from build123d import *

# Parameters (mm, degrees)
F0_W     = 100
F0_H     = 50
F0_R     = 12.5
F1_DEPTH = 10
F2_W     = 10
F2_H     = 50
F3_DEPTH = 5
F5_DEPTH = 50.001
F6_R     = 2.5
F7_DEPTH = 10
F8_R     = 4.99999


# Not quite as in the source:
# - a fillet or chamfer is up to 0.001 mm smaller than in the source, because OpenCascade refuses the exact size


with BuildPart() as f1:
    # F0 (on Top) → F1 (new body)
    with BuildSketch(Plane.XY):
        Rectangle(F0_W, F0_H)
        Circle(F0_R, mode=Mode.SUBTRACT)
    extrude(amount=F1_DEPTH)

    # F2 (on face) → F3 (cut)
    with BuildSketch(Plane.XY.offset(10)):
        with Locations((-35, 0)):
            Rectangle(F2_W, F2_H)
        with BuildLine():
            Line((-7.5, -10), (-7.5, -25))
            Line((-7.5, -25), (7.5, -25))
            Line((7.5, -25), (7.5, -10))
            ThreePointArc((7.5, -10), (0, -12.5), (-7.5, -10))
        make_face()
        with BuildLine():
            Line((7.5, 25), (-7.5, 25))
            Line((-7.5, 25), (-7.5, 10))
            ThreePointArc((-7.5, 10), (0, 12.5), (7.5, 10))
            Line((7.5, 10), (7.5, 25))
        make_face()
    extrude(amount=-F3_DEPTH, mode=Mode.SUBTRACT)

    # F4 (on face) → F5 (cut, through all)
    with BuildSketch(Plane.XZ.offset(25)):
        Polygon((34.8284628647, 10), (19.8284628647, 10), (16.3643612496, 4), (38.2925644799, 4), align=None)
    extrude(amount=-F5_DEPTH, mode=Mode.SUBTRACT)

    # F6 (on face) → F7 (join)
    with BuildSketch(Plane.YZ.offset(50)):
        with Locations((0, 5)):
            Circle(F6_R)
    extrude(amount=F7_DEPTH)

    # F8 (radius 5 in the source; OpenCascade refuses exactly that, so slightly less here)
    f8_edges = [f1.edges().sort_by_distance(p)[0] for p in [
        (-18.75, -25, 10),
        (-18.75, 25, 10),
        (-7.5, -17.5, 10),
        (-7.5, 17.5, 10),
    ]]
    fillet(f8_edges, radius=F8_R)


solid = f1.part
Check sheet for the modelled part. Datum: model origin and axes. Units: mm. A direction names the side the tool comes from. Round coordinates to 2 decimals unless told otherwise and drop trailing zeros. Loops run counter-clockwise (first coordinate to the right, second up) from the corner with the lowest first, then second, coordinate; pieces in that order, holes last. Notation, with made-up numbers: (12, 83) - (48, 83) arc R16 ccw to (48, 105) - close; hole circle Ø6 at (31.25, -2). An arc over 180 degrees is marked (long way). Answer as CSV lines item,"result". Start each with the question number.
Item 1: Release check for a two-part mould opening along X. For faces 1 (the cylindrical face through (-19, -24, 8)), 2 (the flat face through (-45, 0, 10)), 3 (the flat face through (50, 0, 2)) record: +X half, -X half, draft (parallel to the pull), parting line (faces both ways), or undercut.
Item 2: Section check A-A (x = 0). Record the boundary of the cut face in (y, z), and give its area (3 significant figures).
Item 3: Section check D-D (y = 1.5). Record the boundary of the cut face in (x, z).
Item 4: Section check B-B (z = 1.5). Record the boundary of the cut face in (x, y), and give its area (3 significant figures).
Item 5: Depth check by flat-ended pin: P1, Ø5, axis at x = -34.5, y = 3, coming from the +Z side; P2, Ø6, axis at x = 5.5, y = 4.5, coming from the +Z side; P3, Ø1, axis at y = -4.5, z = 7, coming from the +X side. Enter the tip coordinate at first touch or a pass-through.
Item 6: Set-up check for faces 4 (the cylindrical face through (54.93, -0.33, 7.48)), 5 (the flat face through (-1, -25, 4)), 6 (the cylindrical face through (-19, 24, 8)), 7 (the flat face through (27, 0, 4)), 8 (the flat face through (-30, 0, 8)): record each of +Z, -Z, +X, -X, +Y, -Y from which the full face is reachable in a straight line by a thin tool's end or side.
Item 7: Scan lines: line 1 (X direction, y = 8.5, z = 7.25); line 2 (X direction, y = 5.5, z = 6.5); line 3 (Y direction, x = 0, z = 2.5). Record each from-to range of solid material in increasing order. Write a range as [from, to].
Report:
1,face 1,"undercut"
1,face 2,"draft"
1,face 3,"+X half"
2,outline,"(-25, 0) - (-12.5, 0) - (-12.5, 5) - (-25, 5) - close; (12.5, 0) - (25, 0) - (25, 5) - (12.5, 5) - close"
2,area,"125 mm2"
3,outline,"(-50, 0) - (-12.41, 0) - (-12.41, 10) arc R5 ccw to (-12.5, 10) - (-30, 10) - (-30, 5) - (-40, 5) - (-40, 10) - (-50, 10) - close; (12.41, 0) - (50, 0) - (50, 3) - (60, 3) - (60, 7) - (50, 7) - (50, 10) - (34.83, 10) - (38.29, 4) - (16.36, 4) - (19.83, 10) - (12.41, 10) - close"
4,outline,"(-50, -25) - (50, -25) - (50, 25) - (-50, 25) - close; hole circle Ø25 at (0, 0)"
4,area,"4,510 mm2"
5,P1,"stops at z = 5"
5,P2,"passes through"
5,P3,"stops at x = 50"
6,face 4,"+X"
6,face 5,"+Z, -Z, +X, -X, -Y"
6,face 6,"+Z, +Y"
6,face 7,"+Y, -Y"
6,face 8,"+Z, +Y, -Y"
7,line 1,"x = [-50, -40], [-30, -9.17], [9.17, 18.24], [36.42, 50]"
7,line 2,"x = [-50, -40], [-30, -11.22], [11.22, 17.81], [36.85, 50]"
7,line 3,"y = [-25, -12.5], [12.5, 25]"
